The listing builds one solid part. Answer for the finished solid, in the listing's coordinates (mm). Face numbers are marked on the shaded views. A direction names the side the tool comes from. Give positions to 0.01 mm unless a question says otherwise; leave off trailing zeros. Write each loop counter-clockwise with the first axis right and the second up, starting at its lowest first coordinate (ties: lowest second). Pieces come first, ordered by that corner, then holes. Notation, with made-up numbers: M 54,63 L 111,63 A37 cw 111,101 Z; hole C -28,26 d5. An arc over 180 degrees is marked long. Return JSON: item names as keys, results as strings.
from build123d import *

# Parameters (mm, degrees)
SKETCH_1_R      = 21.5
SKETCH_1_R_2    = 1.575
EXTRUDE_1_DEPTH = 3


with BuildPart() as part:
    # 草图1 → 凸台-拉伸1 (new body)
    with BuildSketch(Plane.XY):
        Circle(SKETCH_1_R)
        with Locations((0, 17.5)):
            Circle(SKETCH_1_R_2, mode=Mode.SUBTRACT)
        with Locations((17.5, 0)):
            Circle(SKETCH_1_R_2, mode=Mode.SUBTRACT)
        with Locations((0, -17.5)):
            Circle(SKETCH_1_R_2, mode=Mode.SUBTRACT)
        with Locations((-17.5, 0)):
            Circle(SKETCH_1_R_2, mode=Mode.SUBTRACT)
        with BuildLine():
            ThreePointArc((-5.379173171, 14.989), (-4.428750737, 17.003434709), (-6.443185446, 17.953857143))
            ThreePointArc((-6.443185446, 17.953857143), (-13.488061851, 13.488061851), (-17.953857143, 6.443185446))
            ThreePointArc((-17.953857143, 6.443185446), (-17.003434709, 4.428750737), (-14.989, 5.379173171))
            ThreePointArc((-14.989, 5.379173171), (-11.26067549, 11.26067549), (-5.379173171, 14.989))
        make_face(mode=Mode.SUBTRACT)
        with BuildLine():
            ThreePointArc((5.379173171, 14.989), (11.26067549, 11.26067549), (14.989, 5.379173171))
            ThreePointArc((14.989, 5.379173171), (17.003434709, 4.428750737), (17.953857143, 6.443185446))
            ThreePointArc((17.953857143, 6.443185446), (13.488061851, 13.488061851), (6.443185446, 17.953857143))
            ThreePointArc((6.443185446, 17.953857143), (4.428750737, 17.003434709), (5.379173171, 14.989))
        make_face(mode=Mode.SUBTRACT)
        with BuildLine():
            ThreePointArc((5.379173171, -14.989), (4.428750737, -17.003434709), (6.443185446, -17.953857143))
            ThreePointArc((6.443185446, -17.953857143), (13.488061851, -13.488061851), (17.953857143, -6.443185446))
            ThreePointArc((17.953857143, -6.443185446), (17.003434709, -4.428750737), (14.989, -5.379173171))
            ThreePointArc((14.989, -5.379173171), (11.26067549, -11.26067549), (5.379173171, -14.989))
        make_face(mode=Mode.SUBTRACT)
        with BuildLine():
            ThreePointArc((-5.379173171, -14.989), (-11.26067549, -11.26067549), (-14.989, -5.379173171))
            ThreePointArc((-14.989, -5.379173171), (-17.003434709, -4.428750737), (-17.953857143, -6.443185446))
            ThreePointArc((-17.953857143, -6.443185446), (-13.488061851, -13.488061851), (-6.443185446, -17.953857143))
            ThreePointArc((-6.443185446, -17.953857143), (-4.428750737, -17.003434709), (-5.379173171, -14.989))
        make_face(mode=Mode.SUBTRACT)
    extrude(amount=EXTRUDE_1_DEPTH)


solid = part.part
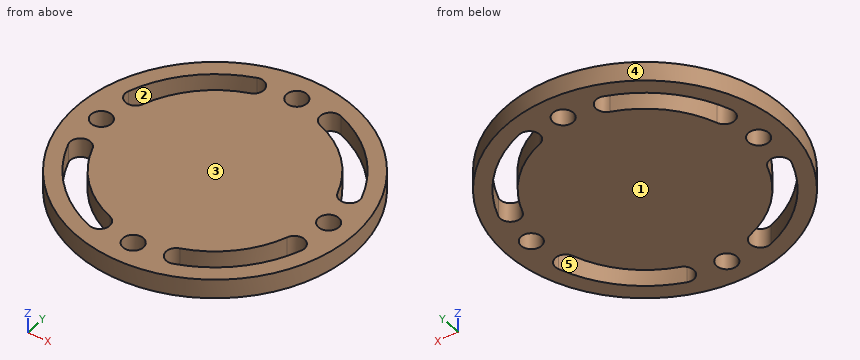
Item 1: Find the intervals of material crossed by line 1 (Y direction, x = 0, z = 1.45) (3 decimals); line 2 (Y direction, x = 8.5, z = 2.05); line 3 (X direction, y = -13, z = 0.85), in increasing order.
Geometry results:
{"line 1": "y = -21.5 to -19.075, -15.925 to 15.925, 19.075 to 21.5", "line 2": "y = -19.75 to -17.08, -13.47 to 13.47, 17.08 to 19.75", "line 3": "x = -17.12 to -13.96, -9.2 to 9.2, 13.96 to 17.12"}
Item 2: A cutting plane is placed at A-A, the plane x = 0. Write down the section's boundary in (y, z) (3 decimals).
Geometry results:
{"outline": "M -21.5,0 L -19.075,0 L -19.075,3 L -21.5,3 Z; M -15.925,0 L 15.925,0 L 15.925,3 L -15.925,3 Z; M 19.075,0 L 21.5,0 L 21.5,3 L 19.075,3 Z"}
Item 3: A cutting plane is placed at C-C, the plane z = 1.7. Count the separate pieces of the cut face and the enclosed holes in it, plus the area to 3 significant figures.
Geometry results:
{"separate pieces": "1", "enclosed holes": "8", "area": "1,200 mm2"}
Item 4: Given pin 1 Ø4 at (x, y) = (0, 17.5) entering from +Z; pin 2 Ø1.5 at (x, z) = (12, 2.5) entering from -Y; pin 3 Ø1.5 at (y, z) = (-3.5, 0.5) entering from +X, each flat-ended and moving along its own axis, determine where each tip first touches the part or whether it passes through.
Geometry results:
{"pin 1": "stops at z = 3", "pin 2": "stops at y = -18.32", "pin 3": "stops at x = 21.32"}
Item 5: Which of the six approach directions +Z, -Z, +X, -X, +Y, -Y give full straight-line access (tool end or side, diameter ignored) to the marked faces 1 and 2?
Geometry results:
{"face 1": "-Z, +X, -X, +Y, -Y", "face 2": "+Z, -Z"}
Item 6: A cutting plane is placed at D-D, the plane y = 16.5. Write down the section's boundary in (x, z).
Geometry results:
{"outline": "M -13.78,0 L -9.57,0 L -9.57,3 L -13.78,3 Z; M -4.34,0 L -1.22,0 L -1.22,3 L -4.34,3 Z; M 1.22,0 L 4.34,0 L 4.34,3 L 1.22,3 Z; M 9.57,0 L 13.78,0 L 13.78,3 L 9.57,3 Z"}
Item 7: Determine the mould class of the marked faces 3, 4 and 5 for opening direction X: +X half, -X half, draft (parallel to the pull), parting line (faces both ways), or undercut.
Geometry results:
{"face 3": "draft", "face 4": "parting line", "face 5": "undercut"}
